The listing builds one solid part. Answer for the finished solid, in the listing's coordinates (mm). Face numbers are marked on the shaded views. A direction names the side the tool comes from. Coordinates: 2 decimals unless noted, no trailing zeros. Loops run counter-clockwise (first coordinate to the right, second up) from the corner with the lowest first, then second, coordinate; pieces in that order, holes last. Notation, with made-up numbers: (11.25, 77) -> (58.25, 77) arc R19 ccw to (58.25, 100) -> close; hole circle Ø7 at (52.5, -18). An arc over 180 degrees is marked (long way). Answer in a Markdown table with one row per item.
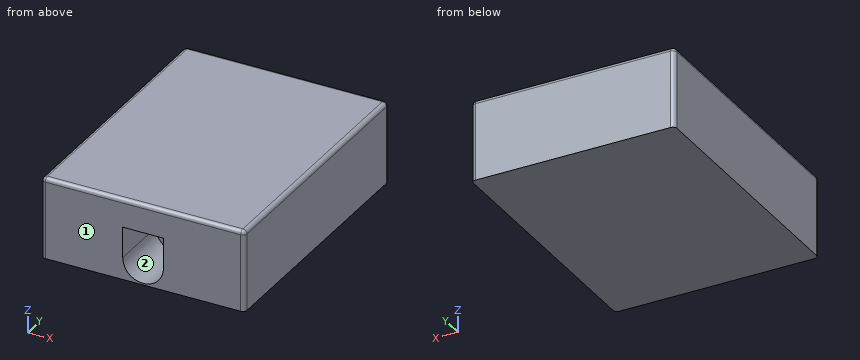
Autodesk Inventor part; units mm, degrees
ref_plane "YZ Plane" through (0, 0, 0) normal (1, 0, 0) x (0, 1, 0)
ref_plane "XZ Plane" through (0, 0, 0) normal (0, 1, 0) x (-1, 0, 0)
ref_plane "XY Plane" through (0, 0, 0) normal (0, 0, 1) x (1, 0, 0)
sketch "Boceto1" plane through (0, 0, 0) normal (0, 0, 1) x (1, 0, 0)
  line L0 (25, -32.5) -> (-25, -32.5)
  line L1 (-25, -32.5) -> (-25, 32.5)
  line L2 (-25, 32.5) -> (25, 32.5)
  line L3 (25, 32.5) -> (25, -32.5)
  line L4 (25, -32.5) -> (-25, 32.5) construction
  line L5 (-25, -32.5) -> (25, 32.5) construction
  point P0 (0, 0)
  dimension "d0" = 50
  dimension "d1" = 65
extrude "Extrusión1" add sketch "Boceto1" along normal blind 20
sketch "Boceto2" plane through (-25, -32.5, 0) normal (0, -1, 0) x (1, 0, 0)
  line L0 (0, 0) -> (0, 20)
  line L1 (0, 13) -> (49.9794, 13)
  line L2 (0, 20) -> (50, 20)
  line L3 (0, 28.5169) -> (0, -2.5169) construction
  line L4 (20, 13) -> (20, 5.4006)
  line L5 (30, 13) -> (30, 5.4006)
  line L6 (25, 0) -> (25, 28.5169) construction
  arc A0 (20, 5.4006) -> (30, 5.4006) centre (25, 5.4006) ccw
  point P0 (0, 13)
  dimension "d4" = 7
  dimension "d5" = 10
  dimension "d6" = 49.9794
  dimension "d7" = 14.5994
  dimension "d8" = 8.5169
  dimension "d9" = 8.5169
extrude "Extrusión2" cut sketch "Boceto2" against normal blind 15
fillet "Empalme1" radius 1 8 edges at (25, 0, 20) (0, 32.5, 20) (25, 32.5, 10) (-25, 0, 20) (-25, 32.5, 10) (0, -32.5, 20) (-25, -32.5, 10) (25, -32.5, 10)
properties part number "componente"
Item 1: A cutting plane is placed at B-B, the plane z = 8. Determine the outline of the cut face in (x, y).
Findings below:
| item | result |
|---|---|
| outline | (-25, -31.5) arc R1 ccw to (-24, -32.5) -> (-5, -32.5) -> (-5, -17.5) -> (5, -17.5) -> (5, -32.5) -> (24, -32.5) arc R1 ccw to (25, -31.5) -> (25, 31.5) arc R1 ccw to (24, 32.5) -> (-24, 32.5) arc R1 ccw to (-25, 31.5) -> close |
Item 2: A tool of negligible diameter and unlimited length cuts with its end or side. For the marked faces 1 and 2, from which of +Z, -Z, +X, -X, +Y, -Y can it reach the whole face along a straight path? Write none if from no direction.
Findings below:
| item | result |
|---|---|
| face 1 | +Z, -Z, +X, -X, -Y |
| face 2 | -Y |
Item 3: A cutting plane is placed at A-A, the plane y = -24.5. Determine the outline of the cut face in (x, z).
Findings below:
| item | result |
|---|---|
| outline | (-25, 0) -> (25, 0) -> (25, 19) arc R1 ccw to (24, 20) -> (-24, 20) arc R1 ccw to (-25, 19) -> close; hole (-5, 5.4) arc R5 ccw to (5, 5.4) -> (5, 13) -> (-5, 13) -> close |
Item 4: A cutting plane is placed at D-D, the plane z = 2.5. Determine the outline of the cut face in (x, y), plus the area to 3 significant figures.
Findings below:
| item | result |
|---|---|
| outline | (-25, -31.5) arc R1 ccw to (-24, -32.5) -> (-4.07, -32.5) -> (-4.07, -17.5) -> (4.07, -17.5) -> (4.07, -32.5) -> (24, -32.5) arc R1 ccw to (25, -31.5) -> (25, 31.5) arc R1 ccw to (24, 32.5) -> (-24, 32.5) arc R1 ccw to (-25, 31.5) -> close |
| area | 3,130 mm2 |
Item 5: A cutting plane is placed at C-C, the plane x = 0. Determine the outline of the cut face in (y, z), plus the area to 3 significant figures.
Findings below:
| item | result |
|---|---|
| outline | (-32.5, 0) -> (32.5, 0) -> (32.5, 19) arc R1 ccw to (31.5, 20) -> (-31.5, 20) arc R1 ccw to (-32.5, 19) -> (-32.5, 13) -> (-17.5, 13) -> (-17.5, 0.4) -> (-32.5, 0.4) -> close |
| area | 1,110 mm2 |
Item 6: Find the intervals of material crossed by probe 1 along X at (y, z) = (-26, 7.75); probe 2 along X at (y, z) = (-27, 4.25); probe 3 along Y at (x, z) = (-2, 11), in increasing order.
Findings below:
| item | result |
|---|---|
| probe 1 | x = -25 to -5, 5 to 25 |
| probe 2 | x = -25 to -4.87, 4.87 to 25 |
| probe 3 | y = -17.5 to 32.5 |
Item 7: A flat-ended cylindrical pin translates along its axis: pin 1 Ø3 at (x, z) = (-0.5, 4) entering from -Y. Find the tip coordinate at first contact, or state that the pin passes through.
Findings below:
| item | result |
|---|---|
| pin 1 | stops at y = -17.5 |
